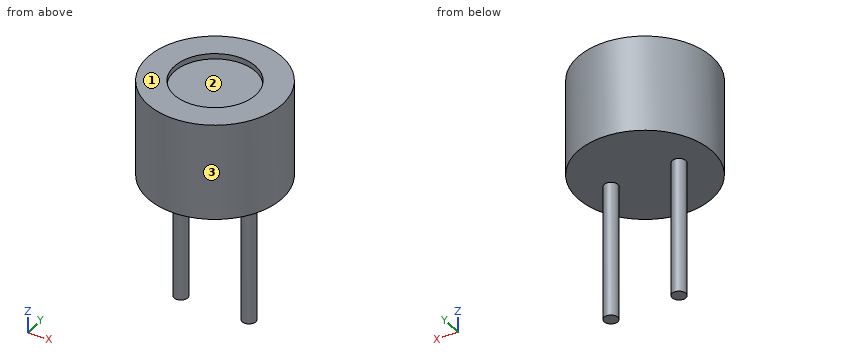
from build123d import *

# Parameters (mm, degrees)
SKETCH_R     = 4.95
PAD_DEPTH    = 7.1
SKETCH001_R  = 0.5
PAD001_DEPTH = 10
SKETCH002_R  = 3
POCKET_DEPTH = 0.4


with BuildPart() as part:
    # Sketch → Pad (new body)
    with BuildSketch(Plane.XY):
        Circle(SKETCH_R)
    extrude(amount=PAD_DEPTH)

    # Sketch001 → Pad001 (new body)
    with BuildSketch(Plane(origin=(0, 0, 0), x_dir=(1, 0, 0), z_dir=(0, 0, -1))):
        with Locations((2.5, 0)):
            Circle(SKETCH001_R)
        with Locations((-2.5, 0)):
            Circle(SKETCH001_R)
    extrude(amount=PAD001_DEPTH)

    # Sketch002 → Pocket (cut)
    with BuildSketch(Plane.XY.offset(7.1)):
        Circle(SKETCH002_R)
    extrude(amount=-POCKET_DEPTH, mode=Mode.SUBTRACT)


solid = part.part
Here's how the part is built. I have some questions about the finished solid (model axes, mm). Face numbers are marked on the shaded views. Round coordinates to 2 decimals unless told otherwise and drop trailing zeros. Write each loop counter-clockwise with the first axis right and the second up, starting at its lowest first coordinate (ties: lowest second). Pieces come first, ordered by that corner, then holes.
1. Suppose I cut it at C-C (y = -0.25). List the corners of the cut face in (x, z) for me, and give its area (3 significant figures).
2. Suppose I cut it at B-B (x = 0). List the corners of the cut face in (y, z) for me, and give its area (3 significant figures).
3. Suppose I cut it at D-D (x = 1.5). List the corners of the cut face in (y, z) for me, and give its area (3 significant figures).
4. Will these pins go through, and if not, where does the flat tip stop? pin 1 Ø3 at (x, y) = (-3, 4) entering from -Z; pin 2 Ø3.5 at (x, y) = (0, 0) entering from +Z.
5. I need wall thicknesses on L1, parallel to Y at x = 0, z = 6.85; L2, parallel to Z at x = 1, y = -3.25; L3, parallel to Z at x = 1, y = 2.25. Which ranges of each line are inside material? Lowest first, please.
6. Suppose I cut it at A-A (z = -2.5). List the corners of the cut face in (x, y) for me, and give its area (3 significant figures).
7. If we mould it in two halves opening along Y, with no side actions, what happens to the marked faces 1, 2 and 3? For each: released by +Y, released by -Y, zero draft, split by the parting line, or undercut.
Answer sheet:
1. outline: (-4.94, 0) - (-2.93, 0) - (-2.93, -10) - (-2.07, -10) - (-2.07, 0) - (2.07, 0) - (2.07, -10) - (2.93, -10) - (2.93, 0) - (4.94, 0) - (4.94, 7.1) - (2.99, 7.1) - (2.99, 6.7) - (-2.99, 6.7) - (-2.99, 7.1) - (-4.94, 7.1) - close
1. area: 85.1 mm2
2. outline: (-4.95, 0) - (4.95, 0) - (4.95, 7.1) - (3, 7.1) - (3, 6.7) - (-3, 6.7) - (-3, 7.1) - (-4.95, 7.1) - close
2. area: 67.9 mm2
3. outline: (-4.72, 0) - (4.72, 0) - (4.72, 7.1) - (2.6, 7.1) - (2.6, 6.7) - (-2.6, 6.7) - (-2.6, 7.1) - (-4.72, 7.1) - close
3. area: 64.9 mm2
4. pin 1: stops at z = 0
4. pin 2: stops at z = 6.7
5. L1: y = -4.95 to -3, 3 to 4.95
5. L2: z = 0 to 7.1
5. L3: z = 0 to 6.7
6. outline: circle Ø1 at (-2.5, 0); circle Ø1 at (2.5, 0)
6. area: 1.57 mm2
7. face 1: zero draft
7. face 2: undercut
7. face 3: split by the parting line
